```python
from build123d import *

# Parameters (mm, degrees)
SKETCH1_W           = 63.5
SKETCH1_H           = 96.52
BOSS_EXTRUDE1_DEPTH = 11.43
FILLET1_R           = 11.43
FILLET2_R           = 3.81
SKETCH2_W           = 12
SKETCH2_H           = 4.49999989
CUT_EXTRUDE1_DEPTH  = 2.54


with BuildPart() as part:
    # Sketch1 → Boss-Extrude1 (new, symmetric)
    with BuildSketch(Plane(origin=(0, 0, 0), x_dir=(1, 0, 0), z_dir=(0, 1, 0))):
        Rectangle(SKETCH1_W, SKETCH1_H)
    extrude(amount=BOSS_EXTRUDE1_DEPTH, both=True)

    # Fillet1
    fillet1_edges = [part.edges().sort_by_distance(p)[0] for p in [
        (-31.75, -11.43, 0),
        (-31.75, 11.43, 0),
        (31.75, -11.43, 0),
        (31.75, 11.43, 0),
    ]]
    fillet(fillet1_edges, radius=FILLET1_R - 0.0001)  # a hair under: the kernel refuses the full size

    # Fillet2
    fillet2_edges = [part.edges().sort_by_distance(p)[0] for p in [
        (0, -11.43, 48.26),
        (0, 11.43, 48.26),
        (28.402259798, 8.082259798, 48.26),
        (28.402259798, -8.082259798, 48.26),
        (-28.402259798, 8.082259798, 48.26),
        (-28.402259798, -8.082259798, 48.26),
        (0, -11.43, -48.26),
        (0, 11.43, -48.26),
        (28.402259798, 8.082259798, -48.26),
        (28.402259798, -8.082259798, -48.26),
        (-28.402259798, 8.082259798, -48.26),
        (-28.402259798, -8.082259798, -48.26),
    ]]
    fillet(fillet2_edges, radius=FILLET2_R)

    # Sketch2 → Cut-Extrude1 (cut)
    with BuildSketch(Plane.XY.offset(48.26)):
        with Locations((-14.32, 0)):
            Rectangle(SKETCH2_W, SKETCH2_H)
    extrude(amount=-CUT_EXTRUDE1_DEPTH, mode=Mode.SUBTRACT)


solid = part.part
```
Design review of the part built by this model. Coordinates are the model's own, in mm. A direction names the side the tool comes from. Coordinates: 2 decimals unless noted, no trailing zeros. One line per question, with ' | ' between items.
(1) Wall thickness on probe 1 along Y at (x, z) = (20.5, -9.5); probe 2 along X at (y, z) = (6.5, 43.5); probe 3 along X at (y, z) = (3, -23.5): over which ranges is each line inside the solid? List them lowest first.
Filled in:
probe 1: y = -11.43 to 11.43 | probe 2: x = -29.72 to 29.72 | probe 3: x = -31.35 to 31.35
(2) Draft analysis for pull direction X (two halves, no side actions). For faces 3 (the face through (-20.32, 0, 47)), 4 (the face through (28.491, -7.993, -0.622)), 5 (the face through (-0.284, 10.284, -47.174)), 6 (the face through (-8.32, 0, 47)), state which applies: released by +X, released by -X, zero draft, split by the parting line, or undercut.
Filled in:
face 3: undercut | face 4: released by +X | face 5: zero draft | face 6: undercut
(3) For pin 1 Ø2 at (y, z) = (-3.5, -28) entering from -X; pin 2 Ø0.8 at (y, z) = (-0.5, 47) entering from +X; pin 3 Ø2 at (x, z) = (-11.5, 47) entering from -Y, all flat-tipped, find the tip position at first contact; note any pin that passes through.
Filled in:
pin 1: stops at x = -31.47 | pin 2: stops at x = 31.07 | pin 3: stops at y = -11.1
(4) Machinability: for faces 1 (the face through (-28.491, 7.993, -0.622)), 2 (the face through (-14, -2.25, 47)), which of the approach directions +Z, -Z, +X, -X, +Y, -Y give a long, thin tool a straight path to every point of the face, cutting with its end or side? Answer none if there is none.
Filled in:
face 1: +Z, -Z, -X, +Y | face 2: +Z
